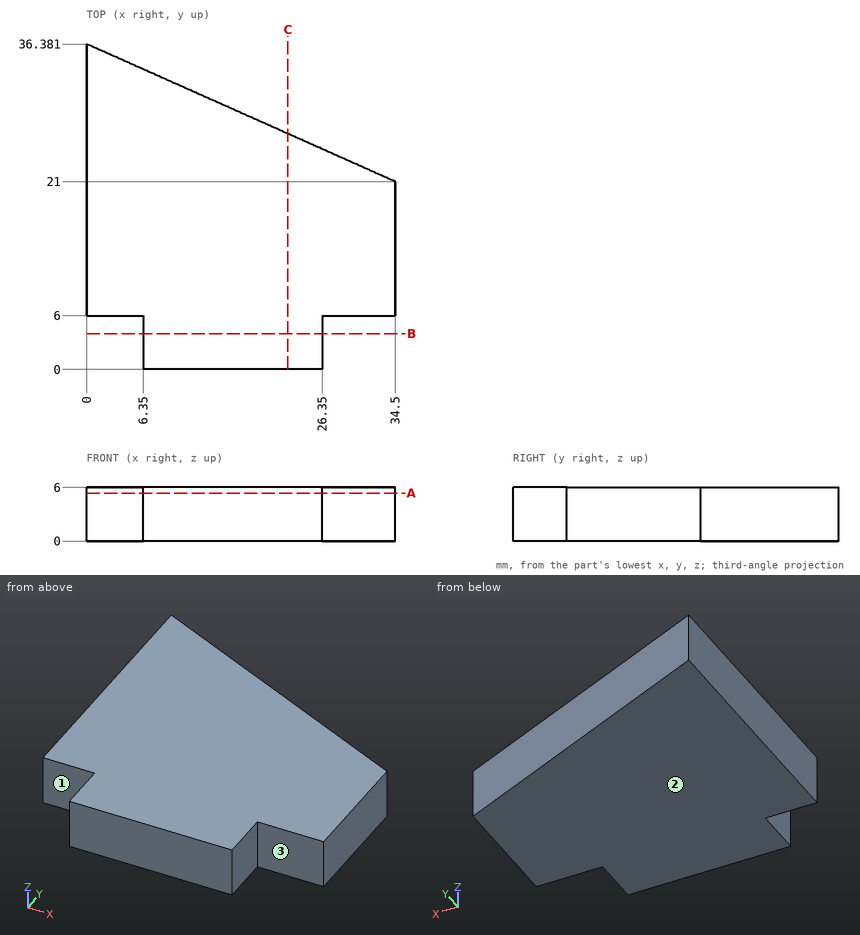
Job drawing, mm, ordinate dimensions from the low corner. One solid piece. A direction names the side the tool comes from. Coordinates: 2 decimals unless noted, no trailing zeros. Order: outer loops, then holes, each group sorted by start corner. A loop starts at its lowest first (then second) coordinate and runs counter-clockwise, first axis right, second up. Notation, with made-up numbers: (30.5, 46.5) -> (45.5, 46.5) arc R22 cw to (45.5, 75.5) -> close; hole circle Ø1 at (60, -4). An arc over 180 degrees is marked (long way). Answer in a Markdown table with one row per item. Add a question column.
Q1. Band-saw the part on C-C, the plane x = 22.5. List the corners of the cut face in (y, z), then the cut area to 3 significant figures.
Q2. Band-saw the part on B-B, the plane y = 4. List the corners of the cut face in (x, z).
Q3. Which spindle directions (+Z, -Z, +X, -X, +Y, -Y) get a long thin tool onto all of the face, cutting with end or side? Do the marked faces 1, 2 and 3. Say none if no direction does.
Q4. Drop flat-ended pins along their axis: pin 1 (3 mm diameter, centred on x = 4.5, z = 2.5, fed in from -Y); pin 2 (1.8 mm diameter, centred on y = 2.5, z = 4, fed in from +X); pin 3 (1 mm diameter, centred on x = 6, z = 2.5, fed in from +Y). Give the stop position or say it passes through.
Q5. Wall check: line 1 along Y through (x, z) = (12.5, 0.65); line 2 along X through (y, z) = (24.5, 2.05); line 3 along Y through (x, z) = (27.5, 4.95). Give the ranges that are in metal, low to high. Write a range as [from, to].
Q6. Band-saw the part on A-A, the plane z = 5.35. List the corners of the cut face in (x, y).
Answers follow:
| question | item | result |
|---|---|---|
| 1 | outline | (0, 0) -> (26.35, 0) -> (26.35, 6) -> (0, 6) -> close |
| 1 | area | 158 mm^2 |
| 2 | outline | (6.35, 0) -> (26.35, 0) -> (26.35, 6) -> (6.35, 6) -> close |
| 3 | face 1 | +Z, -Z, -X, -Y |
| 3 | face 2 | -Z, +X, -X, +Y, -Y |
| 3 | face 3 | +Z, -Z, +X, -Y |
| 4 | pin 1 | y = 6 |
| 4 | pin 2 | x = 26.35 |
| 4 | pin 3 | y = 33.93 |
| 5 | line 1 | [0, 30.81] |
| 5 | line 2 | [0, 26.65] |
| 5 | line 3 | [6, 24.12] |
| 6 | outline | (0, 6) -> (6.35, 6) -> (6.35, 0) -> (26.35, 0) -> (26.35, 6) -> (34.5, 6) -> (34.5, 21) -> (0, 36.38) -> close |
